Work out the finished part from the listing and answer in its coordinate system (mm). A direction names the side the tool comes from. Coordinates: 2 decimals unless noted, no trailing zeros. Loops run counter-clockwise (first coordinate to the right, second up) from the corner with the lowest first, then second, coordinate; pieces in that order, holes last. Notation, with made-up numbers: (15.25, 8.5) -> (54.25, 8.5) arc R32 ccw to (54.25, 34.5) -> close; hole circle Ø9 at (13.25, 81). An arc over 180 degrees is marked (long way). Use a Markdown table: item, result. Add a question column.
```python
from build123d import *

# Parameters (mm, degrees)
SKETCH1_W               = 195.4375
SKETCH1_H               = 97
BOSS_EXTRUDE1_DEPTH     = 65
CUT_EXTRUDE1_DEPTH      = 228.661626996
SKETCH4_W               = 195.4375
SKETCH4_H               = 15
BOSS_EXTRUDE2_DEPTH     = 13.5
BOSS_EXTRUDE3_DEPTH     = 195.4375
SKETCH6_W               = 195.4375
SKETCH6_H               = 2.19
BOSS_EXTRUDE4_DEPTH     = 62
SKETCH7_W               = 195.4375
SKETCH7_H               = 3.24
BOSS_EXTRUDE5_DEPTH     = 22.3
CUT_EXTRUDE2_DEPTH      = 239.145599385
CUT_EXTRUDE2_DEPTH_BACK = 239.145599385
SKETCH8_R               = 1.5


with BuildPart() as part:
    # Sketch1 → Boss-Extrude1 (new body)
    with BuildSketch(Plane(origin=(0, 0, 0), x_dir=(1, 0, 0), z_dir=(0, 1, 0))):
        with Locations((97.71875, 48.5)):
            Rectangle(SKETCH1_W, SKETCH1_H)
    extrude(amount=BOSS_EXTRUDE1_DEPTH)

    # Sketch2 → Cut-Extrude1 (cut, through all)
    with BuildSketch(Plane.ZY):
        Polygon((-97, 65), (-94.65, 6.7), (-89.35, 6.7), (-87, 65), align=None)
        Polygon((-75.16875, 65), (-85.16875, 65), (-82.81875, 6.7), (-77.51875, 6.7), align=None)
        Polygon((-63.3375, 65), (-73.3375, 65), (-70.9875, 6.7), (-65.6875, 6.7), align=None)
        Polygon((-51.50625, 65), (-61.50625, 65), (-59.15625, 6.7), (-53.85625, 6.7), align=None)
        Polygon((-39.675, 65), (-49.675, 65), (-47.325, 6.7), (-42.025, 6.7), align=None)
        Polygon((-27.84375, 65), (-37.84375, 65), (-35.49375, 6.7), (-30.19375, 6.7), align=None)
        Polygon((-16.0125, 65), (-26.0125, 65), (-23.6625, 6.7), (-18.3625, 6.7), align=None)
        Polygon((-4.18125, 65), (-14.18125, 65), (-11.83125, 6.7), (-6.53125, 6.7), align=None)
        Polygon((7.65, 65), (-2.35, 65), (0, 6.7), (5.3, 6.7), align=None)
    extrude(amount=-CUT_EXTRUDE1_DEPTH, mode=Mode.SUBTRACT)

    # Sketch4 → Boss-Extrude2 (add)
    with BuildSketch(Plane(origin=(0, 7, 0), x_dir=(-1, 0, 0), z_dir=(0, -1, 0))):
        with Locations((-97.71875, -6.5)):
            Rectangle(SKETCH4_W, SKETCH4_H)
    extrude(amount=-BOSS_EXTRUDE2_DEPTH)

    # Sketch5 → Boss-Extrude3 (add)
    with BuildSketch(Plane.ZY):
        Polygon((6.265625, 20.5), (7.65, 65), (9.48125, 65), (10.865625, 20.5), align=None)
    extrude(amount=-BOSS_EXTRUDE3_DEPTH)

    # Sketch6 → Boss-Extrude4 (add)
    with BuildSketch(Plane(origin=(0, 6, 0), x_dir=(-1, 0, 0), z_dir=(0, -1, 0))):
        with Locations((-97.71875, 98.095)):
            Rectangle(SKETCH6_W, SKETCH6_H)
    extrude(amount=-BOSS_EXTRUDE4_DEPTH)

    # Sketch7 → Boss-Extrude5 (add)
    with BuildSketch(Plane(origin=(0, 0, -99.19), x_dir=(-1, 0, 0), z_dir=(0, 0, -1))):
        with Locations((-97.71875, 66.38)):
            Rectangle(SKETCH7_W, SKETCH7_H)
    extrude(amount=BOSS_EXTRUDE5_DEPTH)

    # Sketch8 → Cut-Extrude2 (cut, two sides: drawn at the far end of the back side and taken through both)
    with BuildSketch(Plane(origin=(0, 6.7, 0), x_dir=(1, 0, 0), z_dir=(0, 1, 0)).offset(-CUT_EXTRUDE2_DEPTH_BACK)):
        with Locations(Location((190.4375, 92, 0), (0, 0, 270))):
            Circle(SKETCH8_R)
        with Locations(Location((190.4375, -2.85468214, 0), (0, 0, 270))):
            Circle(SKETCH8_R)
        with Locations(Location((5, 92, 0), (0, 0, 90))):
            Circle(SKETCH8_R)
        with Locations(Location((5, -2.85468214, 0), (0, 0, 270))):
            Circle(SKETCH8_R)
    extrude(amount=CUT_EXTRUDE2_DEPTH + CUT_EXTRUDE2_DEPTH_BACK, mode=Mode.SUBTRACT)


solid = part.part
```
Item 1: For a pull along Z with two mould halves and no side action, classify faces 3 (the face through (195.438, 26, -52.8)), 4 (the face through (96.4, 35.4, -52.7)), 5 (the face through (96, 3, 0)) as +Z half, -Z half, draft (parallel to the pull), parting line (faces both ways), or undercut.
Item 2: Section A-A (y = 14.5) is taken. Count the separate pieces of the cut face and the enclosed holes in it, then the cut area to 3 significant figures.
Item 3: Find the intervals of material crossed by probe 1 along X at (y, z) = (5, -92); probe 2 along Y at (x, z) = (147.5, -34); probe 3 along Y at (x, z) = (133.5, -27), in increasing order.
Item 4: Section B-B (z = -32.5) is taken. Determine the outline of the cut face in (x, y), then the cut area to 3 significant figures.
Item 5: Given pin 1 (15.5 mm diameter, centred on x = 114.5, z = 10.5, fed in from -Y); pin 2 (2.5 mm diameter, centred on x = 190.44, z = -92, fed in from +Y); pin 3 (0.5 mm diameter, centred on x = 118, z = -50.5, fed in from +Y); pin 4 (2.5 mm diameter, centred on x = 89, z = -22, fed in from +Y), each flat-ended and moving along its own axis, determine where each tip first touches the part or whether it passes through.
Item 6: For faces 1 (the face through (96, 6.7, -68)), 2 (the face through (99, 7, 7)), determine the directions among +Z, -Z, +X, -X, +Y, -Y from which every point of the face is accessible in a straight line to the end or side of a thin tool.
Output:
| question | item | result |
|---|---|---|
| 1 | face 3 | draft |
| 1 | face 4 | undercut |
| 1 | face 5 | +Z half |
| 2 | separate pieces | 9 |
| 2 | enclosed holes | 2 |
| 2 | area | 12,800 mm2 |
| 3 | probe 1 | x = 0 to 3.5, 6.5 to 188.94, 191.94 to 195.44 |
| 3 | probe 2 | y = 0 to 6.7 |
| 3 | probe 3 | y = 0 to 65 |
| 4 | outline | (0, 0) -> (195.44, 0) -> (195.44, 6.7) -> (0, 6.7) -> close |
| 4 | area | 1,310 mm2 |
| 5 | pin 1 | stops at y = 7 |
| 5 | pin 2 | passes through |
| 5 | pin 3 | stops at y = 65 |
| 5 | pin 4 | stops at y = 6.7 |
| 6 | face 1 | +X, -X, +Y |
| 6 | face 2 | +Z, +X, -X, -Y |
